from build123d import *

# Parameters (mm, degrees)
F0_R        = 38.1
F1_DEPTH    = 127
F3_DEPTH    = 25.4
F4_T4_DEPTH = 137.1700814202
F4_S5_R     = 38.1
F4_T6_DEPTH = 76


# Not quite as in the source:
# - a fillet or chamfer that OpenCascade refuses, or shapes differently, is made with other operations: its cross-section is extruded or revolved along the edge and cut away or added


with BuildPart() as f1:
    # F0 (on Front) → F1 (new body)
    with BuildSketch(Plane.XZ):
        Circle(F0_R)
    extrude(amount=F1_DEPTH)

    # F2 (on face) → F3 (cut)
    with BuildSketch(Plane.XZ.offset(127)):
        with BuildLine():
            ThreePointArc((5.9175740903, -31.1936662944), (-5.0060402001, -31.3528636892), (-15.3369587331, -27.8000035399))
            Line((-15.3369587331, -27.8000035399), (-19.9380463531, -36.1400046019))
            ThreePointArc((-19.9380463531, -36.1400046019), (-6.5078522601, -40.758722796), (7.6928463174, -40.5517661827))
            Line((7.6928463174, -40.5517661827), (5.9175740903, -31.1936662944))
        make_face()
    extrude(amount=-F3_DEPTH, mode=Mode.SUBTRACT)

    # F4: chamfer of 25.4 x 22.86 on 1 edges, made by hand


with BuildPart() as f4_tool2:
    # F4_s3 → F4_t4 (new body)
    with BuildSketch(Plane(origin=(19.2922310235, 0, -101.6963045048), x_dir=(0, 1, 0), z_dir=(-0.1863802863, 0, 0.9824776786))):
        Polygon((-127, 0), (-101.6, 22.86), (-101.6, 0), align=None)
    extrude(amount=F4_T4_DEPTH)

    # F4_s5 → F4_t6 (intersect, symmetric)
    with BuildSketch(Plane.XZ.offset(114.3)):
        Circle(F4_S5_R)
    extrude(amount=F4_T6_DEPTH, both=True, mode=Mode.INTERSECT)

    split(bisect_by=Plane.XZ.offset(127), keep=Keep.BOTTOM)


with BuildPart() as f1_1:
    add(f1.part)

    # F4_t1: union F4_tool2
    add(f4_tool2.part)


solid = f1_1.part
Geometry: final body of the model. Coordinates: model frame, mm. A direction names the side the tool comes from. Give positions to 0.01 mm unless a question says otherwise; leave off trailing zeros. Order: outer loops, then holes, each group sorted by start corner. A loop starts at its lowest first (then second) coordinate and runs counter-clockwise, first axis right, second up. Notation, with made-up numbers: (45.5, 21.5) -> (62.5, 21.5) arc R29 ccw to (62.5, 52.5) -> close; hole circle Ø11 at (18.25, 19). An arc over 180 degrees is marked (long way). Answer as a JSON object with one key per item and string values.
Q1. First-contact query: pin 1 (6 mm diameter, centred on x = 20.5, y = -92.5, fed in from -Z); pin 2 (5 mm diameter, centred on x = 5, y = -46.5, fed in from +Z); pin 3 (4 mm diameter, centred on x = -16.5, y = -29.5, fed in from -Z). Flat tips, straight axial feed; report the tip coordinate or a pass-through.
Entries:
{"pin 1": "stops at z = -33.84", "pin 2": "stops at z = 38.02", "pin 3": "stops at z = -35.23"}
Q2. Access query for faces 1 (the flat face through (-1, -127, 1)), 2 (the cylindrical face through (-7.25, -118.41, -30.91)). Directions: +Z, -Z, +X, -X, +Y, -Y. A direction counts if a zero-diameter tool reaches every point of the face in a straight line with its end or side. Return the directions, or none.
Entries:
{"face 1": "+Z, -Z, +X, -X, -Y", "face 2": "-Z, -Y"}
Q3. Section B-B (x = 14.5). Output: boundary loops of the cut face in (y, z).
Entries:
{"outline": "(-127, -35.23) -> (0, -35.23) -> (0, 35.23) -> (-127, 35.23) -> close"}
Q4. Draft query along X for faces 3 (the flat face through (-16.85, -114.48, -30.54)), 4 (the flat face through (-1, 0, 1)). Return one class per face: released by +X, released by -X, zero draft, split by the parting line, or undercut.
Entries:
{"face 3": "undercut", "face 4": "zero draft"}
Q5. Material intervals for probe 1 along X at (y, z) = (-35.5, -23.5); probe 2 along Z at (x, y) = (20, -8); probe 3 along Z at (x, y) = (11, -87.5), sorted ascending.
Entries:
{"probe 1": "x = -29.99 to 29.99", "probe 2": "z = -32.43 to 32.43", "probe 3": "z = -36.48 to 36.48"}
Q6. Section C-C (z = -25). Output: boundary loops of the cut face in (x, y), plus the area to 3 significant figures.
Entries:
{"outline": "(-28.75, -127) -> (28.75, -127) -> (28.75, 0) -> (-28.75, 0) -> close", "area": "7,300 mm^2"}
Q7. Section A-A (y = -92). Output: boundary loops of the cut face in (x, z).
Entries:
{"outline": "circle Ø76.2 at (0, 0)"}
Q8. Section D-D (y = -115). Output: boundary loops of the cut face in (x, z).
Entries:
{"outline": "(-18.4, -33.36) -> (-15.34, -27.8) arc R31.75 ccw to (-5.05, -31.35) -> (-3.8, -37.91) arc R38.1 ccw (long way) to start"}
